Print and shaded views of the part. All mm, measured from the part's lowest x, y and z. Coordinates: 2 decimals unless noted, no trailing zeros. Order: outer loops, then holes, each group sorted by start corner. A loop starts at its lowest first (then second) coordinate and runs counter-clockwise, first axis right, second up.
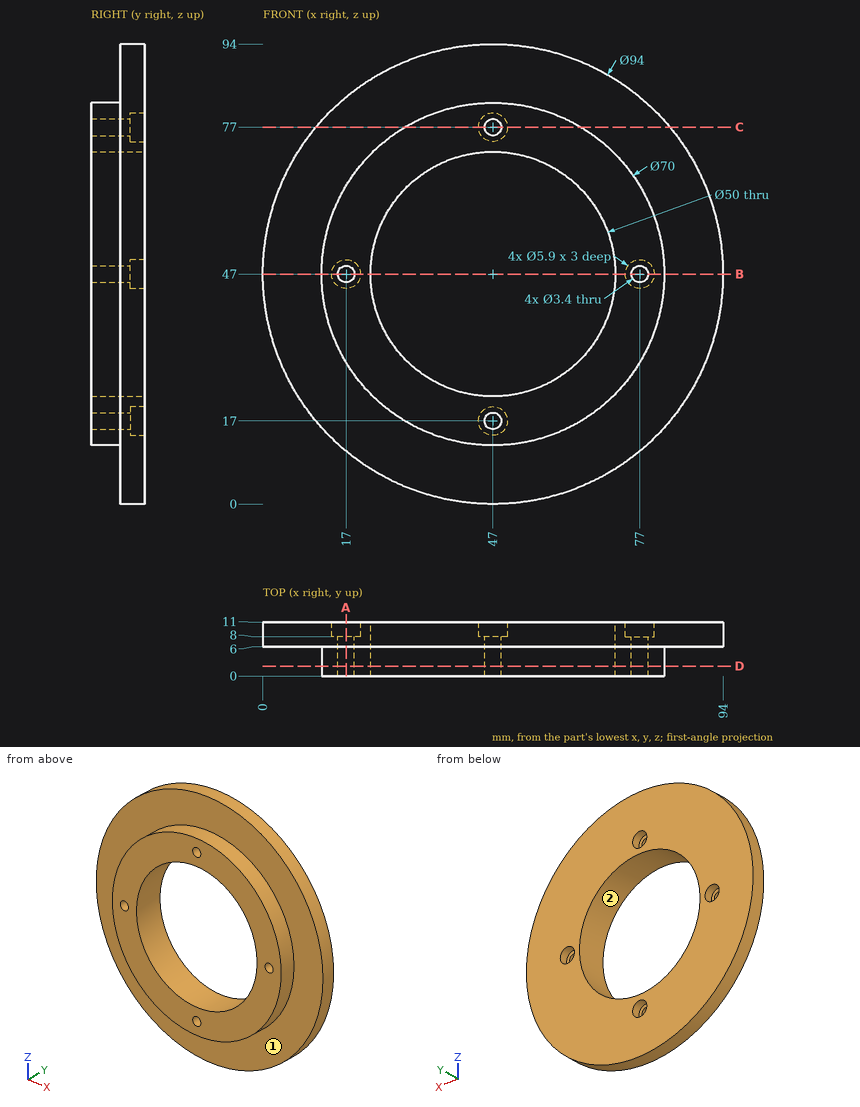
Q1. Probe line 1 (X direction, y = 2.5, z = 47); line 2 (Z direction, x = 47, y = 9.25); line 3 (X direction, y = 5.5, z = 45.5). List the from-to ranges inside material, lowest first.
Established:
line 1: x = 12 to 15.3, 18.7 to 22, 72 to 75.3, 78.7 to 82
line 2: z = 0 to 14.05, 19.95 to 22, 72 to 74.05, 79.95 to 94
line 3: x = 12.03 to 16.2, 17.8 to 22.05, 71.95 to 76.2, 77.8 to 81.97
Q2. Cut at B-B, the plane z = 47. List the corners of the cut face in (x, y), plus the area to 3 significant figures.
Established:
outline: (0, 6) - (12, 6) - (12, 0) - (15.3, 0) - (15.3, 8) - (14.05, 8) - (14.05, 11) - (0, 11) - close; (18.7, 0) - (22, 0) - (22, 11) - (19.95, 11) - (19.95, 8) - (18.7, 8) - close; (72, 0) - (75.3, 0) - (75.3, 8) - (74.05, 8) - (74.05, 11) - (72, 11) - close; (78.7, 0) - (82, 0) - (82, 6) - (94, 6) - (94, 11) - (79.95, 11) - (79.95, 8) - (78.7, 8) - close
area: 250 mm2
Q3. Cut at A-A, the plane x = 17. List the corners of the cut face in (y, z).
Established:
outline: (0, 28.97) - (6, 28.97) - (6, 10.82) - (11, 10.82) - (11, 44.05) - (8, 44.05) - (8, 45.3) - (0, 45.3) - close; (0, 48.7) - (8, 48.7) - (8, 49.95) - (11, 49.95) - (11, 83.18) - (6, 83.18) - (6, 65.03) - (0, 65.03) - close
Q4. Mould opens along X. For the marked faces 1 and 2 say: pulls with the +X half, pulls with the -X half, needs draft (parallel to the pull), parting line crosses it, or undercut.
Established:
face 1: needs draft
face 2: undercut
Q5. Cut at C-C, the plane z = 77. List the corners of the cut face in (x, y).
Established:
outline: (10.82, 6) - (28.97, 6) - (28.97, 0) - (45.3, 0) - (45.3, 8) - (44.05, 8) - (44.05, 11) - (10.82, 11) - close; (48.7, 0) - (65.03, 0) - (65.03, 6) - (83.18, 6) - (83.18, 11) - (49.95, 11) - (49.95, 8) - (48.7, 8) - close
Q6. Drop flat-ended pins along their axis: P1, Ø5.5, axis at x = 47, z = 17, coming from the +Y side; P2, Ø2.5, axis at x = 17, z = 47, coming from the -Y side; P3, Ø2, axis at x = 50.5, y = 1.5, coming from the +Z side; P4, Ø1, axis at y = 6, z = 27, coming from the +X side. Give the stop position or say it passes through.
Established:
P1: stops at y = 8
P2: passes through
P3: stops at z = 81.91
P4: stops at x = 89.76
Q7. Cut at D-D, the plane y = 2. List the corners of the cut face in (x, z).
Established:
outline: circle Ø70 at (47, 47); hole circle Ø3.4 at (17, 47); hole circle Ø50 at (47, 47); hole circle Ø3.4 at (47, 17); hole circle Ø3.4 at (47, 77); hole circle Ø3.4 at (77, 47)
